Design review of the part shown in the three views and the two pictorial views. Dimensions are in mm from the part's minimum x, y and z. A direction names the side the tool comes from. Coordinates: 2 decimals unless noted, no trailing zeros. Write each loop counter-clockwise with the first axis right and the second up, starting at its lowest first coordinate (ties: lowest second). Pieces come first, ordered by that corner, then holes. Notation, with made-up numbers: (51.25, 2) - (66.25, 2) arc R9 cw to (66.25, 15) - close; hole circle Ø11 at (-4, -9). An arc over 180 degrees is marked (long way). Write each question's results on one line, items separated by ' | '.
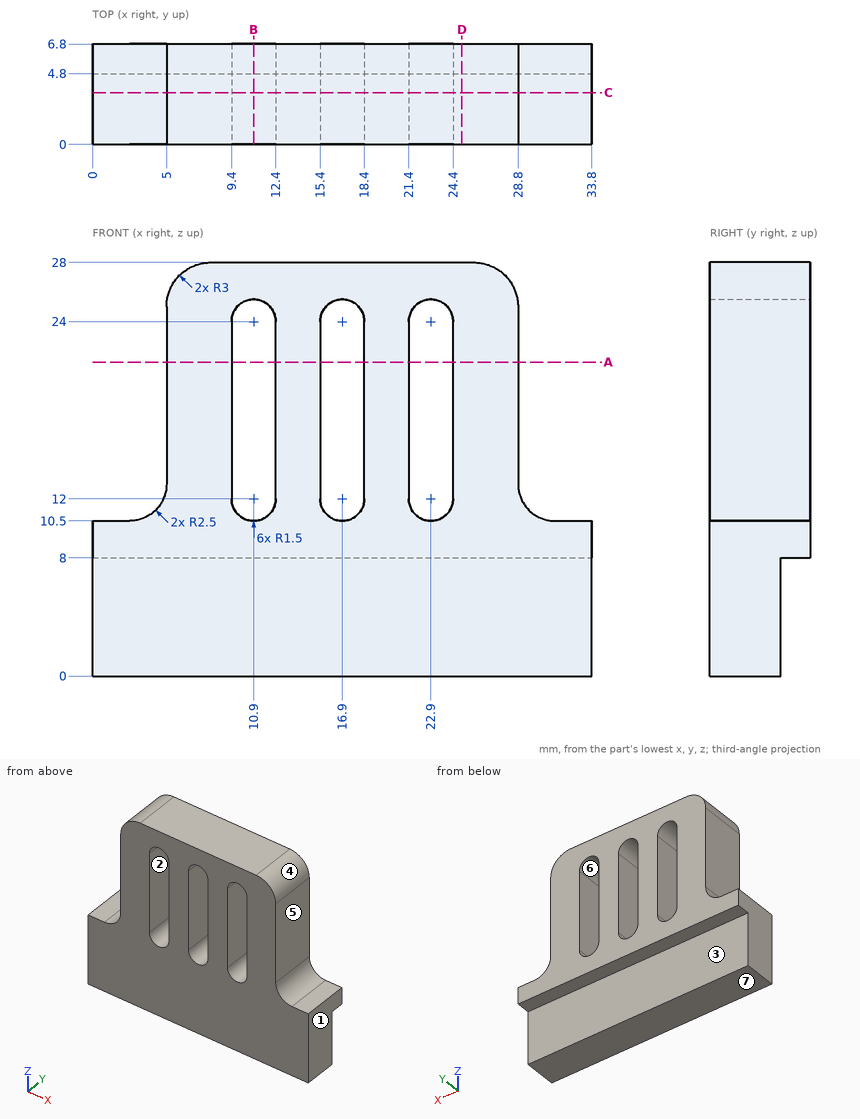
Q1. Mouldability with a two-part tool opening along Z and no side actions: class the marked faces 4, 5, 6 and 7 as pulls with the +Z half, pulls with the -Z half, needs draft (parallel to the pull), parting line crosses it, or undercut.
Results found:
face 4: pulls with the +Z half | face 5: needs draft | face 6: undercut | face 7: pulls with the -Z half
Q2. Take a section at D-D on x = 25. State the section outline as (y, z) points, plus the area to 3 significant figures.
Results found:
outline: (0, 0) - (4.8, 0) - (4.8, 8) - (6.8, 8) - (6.8, 28) - (0, 28) - close | area: 174 mm2
Q3. Take a section at A-A on z = 21.25. State the section outline as (x, y) points, plus the area to 3 significant figures.
Results found:
outline: (5, 0) - (9.4, 0) - (9.4, 6.8) - (5, 6.8) - close; (12.4, 0) - (15.4, 0) - (15.4, 6.8) - (12.4, 6.8) - close; (18.4, 0) - (21.4, 0) - (21.4, 6.8) - (18.4, 6.8) - close; (24.4, 0) - (28.8, 0) - (28.8, 6.8) - (24.4, 6.8) - close | area: 101 mm2
Q4. Take a section at B-B on x = 10.9. State the section outline as (y, z) points.
Results found:
outline: (0, 0) - (4.8, 0) - (4.8, 8) - (6.8, 8) - (6.8, 10.5) - (0, 10.5) - close; (0, 25.5) - (6.8, 25.5) - (6.8, 28) - (0, 28) - close
Q5. Take a section at C-C on y = 3.5. State the section outline as (x, z) points, plus the area to 3 significant figures.
Results found:
outline: (0, 0) - (33.8, 0) - (33.8, 10.5) - (31.3, 10.5) arc R2.5 cw to (28.8, 13) - (28.8, 25) arc R3 ccw to (25.8, 28) - (8, 28) arc R3 ccw to (5, 25) - (5, 13) arc R2.5 cw to (2.5, 10.5) - (0, 10.5) - close; hole (9.4, 12) arc R1.5 ccw to (12.4, 12) - (12.4, 24) arc R1.5 ccw to (9.4, 24) - close; hole (15.4, 12) arc R1.5 ccw to (18.4, 12) - (18.4, 24) arc R1.5 ccw to (15.4, 24) - close; hole (21.4, 12) arc R1.5 ccw to (24.4, 12) - (24.4, 24) arc R1.5 ccw to (21.4, 24) - close | area: 641 mm2
Q6. For the marked faces 1, 2 and 3, list the 3-axis set-ups (+Z, -Z, +X, -X, +Y, -Y) from which the entire face can be reached by the end or side of a thin tool; tool diameter is ignored.
Results found:
face 1: +Z, -Z, +X, +Y, -Y | face 2: +Y, -Y | face 3: -Z, +X, -X, +Y
Q7. Wall thickness on line 1 along X through (y, z) = (5.5, 20); line 2 along Y through (x, z) = (20.5, 3.75); line 3 along Z through (x, y) = (17, 1.25): over which ranges is each line inside the solid? List them lowest first. Write a range as from..to.
Results found:
line 1: 5..9.4, 12.4..15.4, 18.4..21.4, 24.4..28.8 | line 2: 0..4.8 | line 3: 0..10.5, 25.5..28
Q8. For pin 1 (3.5 mm diameter, centred on y = 2, z = 16, fed in from -X); pin 2 (2 mm diameter, centred on y = 3.5, z = 20, fed in from +X); pin 3 (2 mm diameter, centred on x = 2, y = 3.5, fed in from +Z), all flat-tipped, find the tip position at first contact; note any pin that passes through.
Results found:
pin 1: x = 5 | pin 2: x = 28.8 | pin 3: z = 10.55
